Input: part model. Units: mm. Frame: model coordinates. A direction names the side the tool comes from. Round coordinates to 2 decimals unless told otherwise and drop trailing zeros. Order: outer loops, then holes, each group sorted by start corner. A loop starts at its lowest first (then second) coordinate and runs counter-clockwise, first axis right, second up. Notation, with made-up numbers: (-31, 26.5) -> (-10, 26.5) arc R20 ccw to (-10, 42.5) -> close; hole circle Ø3 at (86, 32). An arc over 180 degrees is marked (long way). Use a Markdown table: item, result.
from build123d import *

# Parameters (mm, degrees)
SKETCH1_W           = 73.796067544
SKETCH1_H           = 98.946858939
BOSS_EXTRUDE1_DEPTH = 97
SKETCH2_W           = 45.344140944
SKETCH2_H           = 98.946858939


with BuildPart() as part:
    # Sketch1 → Boss-Extrude1 (new body)
    with BuildSketch(Plane.YZ):
        with Locations((-36.898033772, -49.47342947)):
            Rectangle(SKETCH1_W, SKETCH1_H)
    extrude(amount=BOSS_EXTRUDE1_DEPTH)

    # Sketch2 → Cut-Revolve1 (revolve, cut)
    with BuildSketch(Plane.YZ.offset(97)):
        with Locations((-22.672070472, -49.47342947)):
            Rectangle(SKETCH2_W, SKETCH2_H)
    revolve(axis=Axis((97, 0, -98.946858939), (0, -1, 0)), mode=Mode.SUBTRACT)


solid = part.part
1) Set-up query: faces 1 (the face through (59, -45.344, -60)), 2 (the face through (48, -37, 0)). Return all of +Z, -Z, +X, -X, +Y, -Y with unobstructed straight access to the full face (end or side cutting, diameter ignored); none if empty.
Answer key:
| item | result |
|---|---|
| face 1 | -Z, +X, +Y |
| face 2 | +Z, +X, -X, +Y, -Y |
2) Ray query, probe 1 along Y at (x, z) = (48, -39); probe 2 along X at (y, z) = (-44.5, -63.5); probe 3 along X at (y, z) = (-38.5, -50). Return the intervals inside material, ascending.
Answer key:
| item | result |
|---|---|
| probe 1 | y = -73.8 to -45.34 |
| probe 2 | x = 0 to 4.62 |
| probe 3 | x = 0 to 11.01 |
3) Cut plane C-C on z = -16. Return loops of the section in (x, y).
Answer key:
| item | result |
|---|---|
| outline | (0, -73.8) -> (97, -73.8) -> (97, -45.34) -> (43.05, -45.34) -> (43.05, 0) -> (0, 0) -> close |
4) Cut plane A-A on y = -18.5. Return loops of the section in (x, z).
Answer key:
| item | result |
|---|---|
| outline | (0, -79.42) arc R98.95 cw to (97, 0) -> (0, 0) -> close |
5) Cut plane B-B on x = 40. Return loops of the section in (y, z).
Answer key:
| item | result |
|---|---|
| outline | (-73.8, -98.95) -> (-45.34, -98.95) -> (-45.34, -18.07) -> (0, -18.07) -> (0, 0) -> (-73.8, 0) -> close |
6) Contact query for flat-ended pins moving along their axis: P1, Ø1, axis at x = 67, z = -43.5, coming from the +Y side; P2, Ø3, axis at y = -8, z = -29, coming from the +X side; P3, Ø3, axis at x = 13, z = -30, coming from the +Y side; P4, Ø10, axis at y = -16, z = -82, coming from the +X side. Output: stop coordinate, or through.
Answer key:
| item | result |
|---|---|
| P1 | stops at y = -45.34 |
| P2 | stops at x = 28.55 |
| P3 | stops at y = 0 |
| P4 | stops at x = 0.52 |
